from build123d import *

# Parameters (mm, degrees)
SKETCH1_W                      = 20
SKETCH1_H                      = 40
BOSS_EXTRUDE1_DEPTH            = 10
CUT_EXTRUDE1_START             = -2
CUT_EXTRUDE1_DEPTH             = 23.494897428
CUT_EXTRUDE1_DRAFT             = 1
SKETCH4_R                      = 5.08
BOSS_EXTRUDE2_DEPTH            = 2.54
SKETCH5_R                      = 1.75
CUT_EXTRUDE2_DEPTH             = 24.748684174
CBORE_FOR_M5_SHCS1_D           = 5.5
CBORE_FOR_M5_SHCS1_DEPTH       = 12
CBORE_FOR_M5_SHCS1_CBORE_D     = 10
CBORE_FOR_M5_SHCS1_CBORE_DEPTH = 5
CBORE_FOR_M5_SHCS1_TIP         = 1.652366702
FILLET1_R                      = 3


with BuildPart() as part:
    # Sketch1 → Boss-Extrude1 (new body)
    with BuildSketch(Plane(origin=(0, 0, 0), x_dir=(1, 0, 0), z_dir=(0, 1, 0))):
        Rectangle(SKETCH1_W, SKETCH1_H)
    extrude(amount=BOSS_EXTRUDE1_DEPTH)


with BuildPart() as cut_extrude1_tool:
    # Sketch3 → Cut-Extrude1 (with draft: the straight prism first)
    with BuildSketch(Plane(origin=(0, 10, 0), x_dir=(1, 0, 0), z_dir=(0, 1, 0)).offset(CUT_EXTRUDE1_START)):
        Polygon((3.175426481, 0), (1.58771324, 2.75), (-1.58771324, 2.75), (-3.175426481, 0), (-1.58771324, -2.75), (1.58771324, -2.75), align=None)
    extrude(amount=-CUT_EXTRUDE1_DEPTH)
    # Cut-Extrude1: the draft: its side faces are tilted about the plane it starts from
    cut_extrude1_sides = [cut_extrude1_tool.faces().sort_by_distance(p)[0] for p in [
        (2.38156986, -3.747448714, -1.375),
        (0, -3.747448714, -2.75),
        (-2.38156986, -3.747448714, -1.375),
        (-2.38156986, -3.747448714, 1.375),
        (0, -3.747448714, 2.75),
        (2.38156986, -3.747448714, 1.375),
    ]]
    draft(cut_extrude1_sides, Plane(origin=(0, 10, 0), x_dir=(1, 0, 0), z_dir=(0, 1, 0)).offset(CUT_EXTRUDE1_START), CUT_EXTRUDE1_DRAFT)


with BuildPart() as part_1:
    add(part.part)

    # Cut-Extrude1: cut by cut_extrude1_tool
    add(cut_extrude1_tool.part, mode=Mode.SUBTRACT)

    # Sketch4 → Boss-Extrude2 (add)
    with BuildSketch(Plane(origin=(0, 10, 0), x_dir=(1, 0, 0), z_dir=(0, 1, 0))):
        with Locations(Location((0, 0, 0), (0, 0, 270))):
            Circle(SKETCH4_R)
    extrude(amount=BOSS_EXTRUDE2_DEPTH)

    # Sketch5 → Cut-Extrude2 (cut, through all)
    with BuildSketch(Plane.XZ.offset(-8)):
        with Locations(Location((0, 0, 0), (0, 0, 270))):
            Circle(SKETCH5_R)
    extrude(amount=-CUT_EXTRUDE2_DEPTH, mode=Mode.SUBTRACT)

    # CBORE for M5 SHCS1
    with Locations(Plane(origin=(0, 10, 0), x_dir=(1, 0, 0), z_dir=(0, 1, 0))):
        with Locations((0, -12), (0, 12)):
            CounterBoreHole(CBORE_FOR_M5_SHCS1_D / 2, CBORE_FOR_M5_SHCS1_CBORE_D / 2, CBORE_FOR_M5_SHCS1_CBORE_DEPTH, depth=CBORE_FOR_M5_SHCS1_DEPTH)
            with Locations((0, 0, -(CBORE_FOR_M5_SHCS1_DEPTH + CBORE_FOR_M5_SHCS1_TIP / 2))):  # 118° drill point
                Cone(0, CBORE_FOR_M5_SHCS1_D / 2, CBORE_FOR_M5_SHCS1_TIP, mode=Mode.SUBTRACT)

    # Fillet1
    fillet1_edges = [part_1.edges().sort_by_distance(p)[0] for p in [
        (10, 5, 20),
        (-10, 5, 20),
        (-10, 5, -20),
        (10, 5, -20),
    ]]
    fillet(fillet1_edges, radius=FILLET1_R)


solid = part_1.part
Design review of the part built by this model. Coordinates are the model's own, in mm. A direction names the side the tool comes from. Give positions to 0.01 mm unless a question says otherwise; leave off trailing zeros. Write each loop counter-clockwise with the first axis right and the second up, starting at its lowest first coordinate (ties: lowest second). Pieces come first, ordered by that corner, then holes. Notation, with made-up numbers: M -40,77 L -22,77 A23 ccw -22,106 Z; hole C 62,-30 d1. An arc over 180 degrees is marked long. Return JSON: item names as keys, results as strings. Group by question number.
Item 1: Take a section at B-B (x = 0). Count the separate pieces of the cut face and the enclosed holes in it, plus the area to 3 significant figures.
Item 2: Take a section at A-A (z = 12). Give the boundary of the cut face in (x, y), plus the area to 4 significant figures.
Item 3: Wall thickness on line 1 along Z through (x, y) = (0, 7.95); line 2 along X through (y, z) = (11.6, 0); line 3 along Z through (x, y) = (2.25, 2.25): over which ranges is each line inside the solid? List them lowest first.
Item 4: Take a section at D-D (z = -10). Give the boundary of the cut face in (x, y), plus the area to 3 significant figures.
Item 5: The part is to be moulded in two halves that separate along X. For faces 1 (the cylindrical face through (5.037, 11.252, -0.661)), 2 (the cylindrical face through (-0.651, 7.535, 7.043)), 3 (the flat face through (-2, 10, -5)), say which applies: pulls with the +X half, pulls with the -X half, needs draft (parallel to the pull), parting line crosses it, or undercut.
Item 6: Take a section at C-C (y = 9.5). Give the boundary of the cut face in (x, z), plus the area to 3 significant figures.
Item 7: Tool access review of faces 4 (the flat face through (2.2, 5, -9.8)), 5 (the flat face through (0, 5, -20)): name each direction out of +Z, -Z, +X, -X, +Y, -Y from which nothing blocks a thin tool from reaching the whole face with its end or side.
Item 8: Clearance check with flat-ended pins moving along their axes: pin 1 Ø1.5 at (x, z) = (-2.5, -13.5) entering from -Y; pin 2 Ø8 at (x, z) = (0, 9.5) entering from +Y; pin 3 Ø4.5 at (x, z) = (0, -12) entering from +Y; pin 4 Ø7 at (x, z) = (0, 12) entering from +Y. State where each tip first meets the part, or that it passes through.
Return value:
{
 "1": {"separate pieces": "4", "enclosed holes": "0", "area": "210 mm2"},
 "2": {"outline": "M -10,0 L -2.75,0 L -2.75,5 L -5,5 L -5,10 L -10,10 Z; M 2.75,0 L 10,0 L 10,10 L 5,10 L 5,5 L 2.75,5 Z", "area": "122.5 mm2"},
 "3": {"line 1": "z = -20 to -17, -7 to -2.75, 2.75 to 7, 17 to 20", "line 2": "x = -5.08 to -1.75, 1.75 to 5.08", "line 3": "z = -20 to -13.58, -10.42 to -1.8, 1.8 to 10.42, 13.58 to 20"},
 "4": {"outline": "M -10,0 L -1.89,0 L -1.89,5 L -4.58,5 L -4.58,10 L -10,10 Z; M 1.89,0 L 10,0 L 10,10 L 4.58,10 L 4.58,5 L 1.89,5 Z", "area": "135 mm2"},
 "5": {"face 1": "parting line crosses it", "face 2": "undercut", "face 3": "needs draft"},
 "6": {"outline": "M -10,-17 A3 ccw -7,-20 L 7,-20 A3 ccw 10,-17 L 10,17 A3 ccw 7,20 L -7,20 A3 ccw -10,17 Z; hole C 0,-12 d10; hole C 0,12 d10; hole C 0,0 d3.5", "area": "626 mm2"},
 "7": {"face 4": "+Y", "face 5": "-Z, +X, -X, +Y, -Y"},
 "8": {"pin 1": "stops at y = 0", "pin 2": "stops at y = 10", "pin 3": "passes through", "pin 4": "stops at y = 5"}
}
